from build123d import *

# Parameters (mm, degrees)
BOSS_EXTRU_1_DEPTH      = 3
CONG_8_R                = 25
D_GAGEMENT_M31_D        = 3.4
ENL_V_MAT_EXTRU_1_DEPTH = 154.69791124
D_GAGEMENT_M35_D        = 3.4
D_GAGEMENT_M35_DEPTH    = 7
D_GAGEMENT_M35_TIP      = 1.021463052


with BuildPart() as part:
    # Esquisse1 → Boss.-Extru.1 (new body)
    with BuildSketch(Plane(origin=(0, 0, 0), x_dir=(1, 0, 0), z_dir=(0, 1, 0))):
        Polygon((-102.5, 59.178402592), (-102.5, -59.178402592), (0, -118.356805184), (102.5, -59.178402592), (102.5, 59.178402592), (0, 118.356805184), align=None)
    extrude(amount=BOSS_EXTRU_1_DEPTH)

    # Congé8
    cong_8_edges = [part.edges().sort_by_distance(p)[0] for p in [
        (0, 1.5, -118.356805184),
        (102.5, 1.5, -59.178402592),
        (102.5, 1.5, 59.178402592),
        (0, 1.5, 118.356805184),
        (-102.5, 1.5, 59.178402592),
        (-102.5, 1.5, -59.178402592),
    ]]
    fillet(cong_8_edges, radius=CONG_8_R)

    # Dégagement M31 (through all)
    with Locations(Plane(origin=(0, 3, 0), x_dir=(1, 0, 0), z_dir=(0, 1, 0))):
        with Locations((57.1, 22.9999993), (48.1, 22.9999993), (52.6, 22.9999993), (-52.6, 22.9999993), (-48.1, 22.9999993), (-57.1, 22.9999993), (-127.319090426, 28.910605245)):
            Hole(D_GAGEMENT_M31_D / 2)

    # Esquisse4 → Enlèv. mat.-Extru.1 (cut, through all)
    with BuildSketch(Plane(origin=(0, 3, 0), x_dir=(1, 0, 0), z_dir=(0, 1, 0))):
        with BuildLine():
            Line((-55, -9.372115214), (-55, -12.372115214))
            ThreePointArc((-55, -12.372115214), (-53.5, -13.872115214), (-52, -12.372115214))
            Line((-52, -12.372115214), (-52, -9.372115214))
            ThreePointArc((-52, -9.372115214), (-53.5, -7.872115214), (-55, -9.372115214))
        make_face()
        with BuildLine():
            Line((-55, -32.872115214), (-55, -35.872115214))
            ThreePointArc((-55, -35.872115214), (-53.5, -37.372115214), (-52, -35.872115214))
            Line((-52, -35.872115214), (-52, -32.872115214))
            ThreePointArc((-52, -32.872115214), (-53.5, -31.372115214), (-55, -32.872115214))
        make_face()
        with BuildLine():
            Line((55, -9.372115214), (55, -12.372115214))
            ThreePointArc((55, -12.372115214), (53.5, -13.872115214), (52, -12.372115214))
            Line((52, -12.372115214), (52, -9.372115214))
            ThreePointArc((52, -9.372115214), (53.5, -7.872115214), (55, -9.372115214))
        make_face()
        with BuildLine():
            Line((55, -32.872115214), (55, -35.872115214))
            ThreePointArc((55, -35.872115214), (53.5, -37.372115214), (52, -35.872115214))
            Line((52, -35.872115214), (52, -32.872115214))
            ThreePointArc((52, -32.872115214), (53.5, -31.372115214), (55, -32.872115214))
        make_face()
    extrude(amount=-ENL_V_MAT_EXTRU_1_DEPTH, mode=Mode.SUBTRACT)

    # Dégagement M35
    with Locations(Plane(origin=(0, 3, 0), x_dir=(1, 0, 0), z_dir=(0, 1, 0))):
        with Locations((-90.594469683, -27.994469683), (-8.9, -35.75), (8.9, -35.75), (0, -109.639291724), (90.594469683, -27.994469683), (98.85, -27.55), (98.75, 32.45), (98.75, 40.25), (15.43813191, 105.113468551), (-15.43813191, 105.113468551), (-98.75, 32.45), (-98.75, 40.25)):
            Hole(D_GAGEMENT_M35_D / 2, depth=D_GAGEMENT_M35_DEPTH)
            with Locations((0, 0, -(D_GAGEMENT_M35_DEPTH + D_GAGEMENT_M35_TIP / 2))):  # 118° drill point
                Cone(0, D_GAGEMENT_M35_D / 2, D_GAGEMENT_M35_TIP, mode=Mode.SUBTRACT)


solid = part.part
Model file for the job. Use its own axes, mm. Round coordinates to 2 decimals unless told otherwise and drop trailing zeros. Write each question's results on one line, items separated by ' | '. Start each with the question number.
(1) Saw through at A-A, the plane y = 0.8. State how many separate pieces and enclosed holes the cut face has, then the cut area to 3 significant figures.
(2) Drop a flat-ended pin along its axis: pin 1 (3 mm diameter, centred on x = 98.75, z = -32.45, fed in from -Y). Give the stop position or say it passes through.
(3) Probe probe 1 along X at (y, z) = (1.75, 35.75); probe 2 along X at (y, z) = (0.8, 27.55); probe 3 along X at (y, z) = (1.75, -40.25). List the from-to ranges inside material, lowest first. Write a range as from..to.
Established:
1) separate pieces: 1 | enclosed holes: 22 | area: 36,000 mm^2
2) pin 1: passes through
3) probe 1: x = -102.5..-55, -52..-10.6, -7.2..7.2, 10.6..52, 55..102.5 | probe 2: x = -102.5..-92.24, -88.95..88.95, 92.24..97.15, 100.55..102.5 | probe 3: x = -102.5..-100.45, -97.05..97.05, 100.45..102.5
